```python
from build123d import *

# Parameters (mm, degrees)
SKETCH1_W           = 2.9972
SKETCH1_H           = 19.05
BOSS_EXTRUDE1_DEPTH = 2.9972


with BuildPart() as part:
    # Sketch1 → Boss-Extrude1 (new body)
    with BuildSketch(Plane.XY):
        Polygon((-12.4968, 0), (-12.4968, -2.9972), (-29.0068, -2.9972), (-29.0068, -383.9972), (-26.8986, -383.9972), (-26.8986, -364.9472), (-23.9014, -364.9472), (-23.9014, -383.9972), (-12.4968, -383.9972), (-12.4968, -386.9944), (12.4206, -386.9944), (12.4206, -383.9972), (23.9014, -383.9972), (23.9014, -364.9472), (26.8986, -364.9472), (26.8986, -383.9972), (28.9306, -383.9972), (28.9306, -2.9972), (12.4206, -2.9972), (12.4206, 0), align=None)
        with Locations((-25.4, -349.0722)):
            Rectangle(SKETCH1_W, SKETCH1_H, mode=Mode.SUBTRACT)
        with Locations((-25.4, -323.6722)):
            Rectangle(SKETCH1_W, SKETCH1_H, mode=Mode.SUBTRACT)
        with Locations((-25.4, -298.2722)):
            Rectangle(SKETCH1_W, SKETCH1_H, mode=Mode.SUBTRACT)
        with Locations((-25.4, -272.8722)):
            Rectangle(SKETCH1_W, SKETCH1_H, mode=Mode.SUBTRACT)
        with Locations((-25.4, -247.4722)):
            Rectangle(SKETCH1_W, SKETCH1_H, mode=Mode.SUBTRACT)
        with Locations((-25.4, -222.0722)):
            Rectangle(SKETCH1_W, SKETCH1_H, mode=Mode.SUBTRACT)
        with Locations((-25.4, -196.6722)):
            Rectangle(SKETCH1_W, SKETCH1_H, mode=Mode.SUBTRACT)
        with Locations((25.4, -349.0722)):
            Rectangle(SKETCH1_W, SKETCH1_H, mode=Mode.SUBTRACT)
        with Locations((25.4, -323.6722)):
            Rectangle(SKETCH1_W, SKETCH1_H, mode=Mode.SUBTRACT)
        with Locations((25.4, -298.2722)):
            Rectangle(SKETCH1_W, SKETCH1_H, mode=Mode.SUBTRACT)
        with Locations((25.4, -272.8722)):
            Rectangle(SKETCH1_W, SKETCH1_H, mode=Mode.SUBTRACT)
        with Locations((25.4, -247.4722)):
            Rectangle(SKETCH1_W, SKETCH1_H, mode=Mode.SUBTRACT)
        with Locations((25.4, -222.0722)):
            Rectangle(SKETCH1_W, SKETCH1_H, mode=Mode.SUBTRACT)
        with Locations((25.4, -196.6722)):
            Rectangle(SKETCH1_W, SKETCH1_H, mode=Mode.SUBTRACT)
        with Locations((-25.4, -171.2722)):
            Rectangle(SKETCH1_W, SKETCH1_H, mode=Mode.SUBTRACT)
        with Locations((-25.4, -145.8722)):
            Rectangle(SKETCH1_W, SKETCH1_H, mode=Mode.SUBTRACT)
        with Locations((-25.4, -120.4722)):
            Rectangle(SKETCH1_W, SKETCH1_H, mode=Mode.SUBTRACT)
        with Locations((-25.4, -95.0722)):
            Rectangle(SKETCH1_W, SKETCH1_H, mode=Mode.SUBTRACT)
        with Locations((-25.4, -69.6722)):
            Rectangle(SKETCH1_W, SKETCH1_H, mode=Mode.SUBTRACT)
        with Locations((-25.4, -44.2722)):
            Rectangle(SKETCH1_W, SKETCH1_H, mode=Mode.SUBTRACT)
        with Locations((-25.4, -18.8722)):
            Rectangle(SKETCH1_W, SKETCH1_H, mode=Mode.SUBTRACT)
        with Locations((25.4, -171.2722)):
            Rectangle(SKETCH1_W, SKETCH1_H, mode=Mode.SUBTRACT)
        with Locations((25.4, -145.8722)):
            Rectangle(SKETCH1_W, SKETCH1_H, mode=Mode.SUBTRACT)
        with Locations((25.4, -120.4722)):
            Rectangle(SKETCH1_W, SKETCH1_H, mode=Mode.SUBTRACT)
        with Locations((25.4, -95.0722)):
            Rectangle(SKETCH1_W, SKETCH1_H, mode=Mode.SUBTRACT)
        with Locations((25.4, -69.6722)):
            Rectangle(SKETCH1_W, SKETCH1_H, mode=Mode.SUBTRACT)
        with Locations((25.4, -44.2722)):
            Rectangle(SKETCH1_W, SKETCH1_H, mode=Mode.SUBTRACT)
        with Locations((25.4, -18.8722)):
            Rectangle(SKETCH1_W, SKETCH1_H, mode=Mode.SUBTRACT)
    extrude(amount=BOSS_EXTRUDE1_DEPTH)


solid = part.part
```
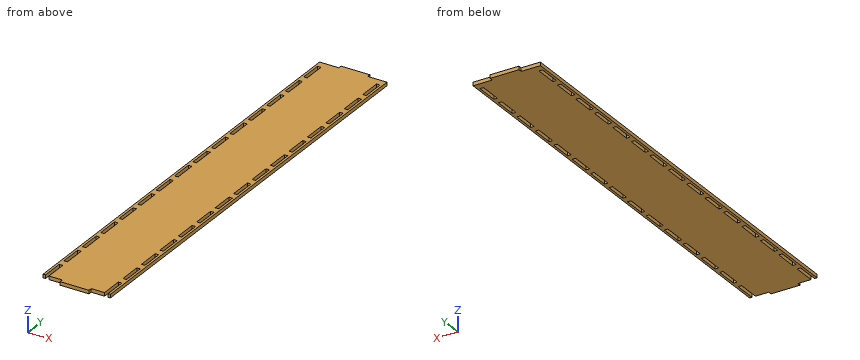
For this review, take the finished solid that the model builds, in its own axes (mm). Coordinates: 2 decimals unless noted, no trailing zeros. Order: outer loops, then holes, each group sorted by start corner. A loop starts at its lowest first (then second) coordinate and runs counter-clockwise, first axis right, second up. Notation, with made-up numbers: (-30, -14.75) - (12, -14.75) arc R23 cw to (12, 5.25) - close; hole circle Ø2 at (-20.5, 88). An arc over 180 degrees is marked (long way). Answer as a JSON object with one key per item and string values. Group by question number.
1. We need section A-A on y = -198.5. State the section outline as (x, z) points, then the cut area to 3 significant figures.
2. Clearance check with flat-ended pins moving along their axes: P1, Ø0.9, axis at x = 25, z = 1, coming from the -Y side; P2, Ø1.5, axis at x = -25.5, z = 1.5, coming from the +Y side; P3, Ø1.7, axis at x = -28, z = 1.5, coming from the -Y side; P4, Ø5, axis at x = -11.5, y = -311, coming from the -Z side. State where each tip first meets the part, or that it passes through.
3. We need section B-B on z = 1.8. Give the number of separate pieces and of enclosed holes in the cut face, then the cut area to 3 significant figures.
4. We need section C-C on x = -19. State the section outline as (y, z) points, then the cut area to 3 significant figures.
5. For probe 1 along X at (y, z) = (-292, 0.4); probe 2 along Y at (x, z) = (17, 2.2), list the stretches that pass through material, from the lowest coordinate up.
Final values:
{
 "1": {"outline": "(-29.01, 0) - (-26.9, 0) - (-26.9, 3) - (-29.01, 3) - close; (-23.9, 0) - (23.9, 0) - (23.9, 3) - (-23.9, 3) - close; (26.9, 0) - (28.93, 0) - (28.93, 3) - (26.9, 3) - close", "area": "156 mm²"},
 "2": {"P1": "y = -364.95", "P2": "y = -3", "P3": "y = -384", "P4": "z = 0"},
 "3": {"separate pieces": "1", "enclosed holes": "28", "area": "20,500 mm²"},
 "4": {"outline": "(-384, 0) - (-3, 0) - (-3, 3) - (-384, 3) - close", "area": "1,140 mm²"},
 "5": {"probe 1": "-29.01 to -26.9, -23.9 to 23.9, 26.9 to 28.93", "probe 2": "-384 to -3"}
}
